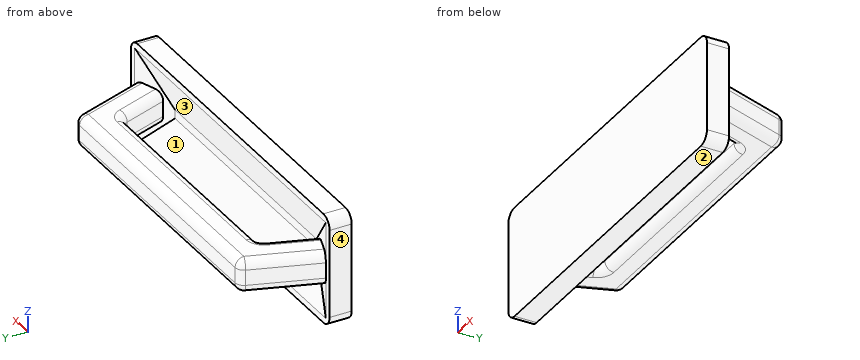
```python
from build123d import *

# Parameters (mm, degrees)
SKETCH1_W                = 160
SKETCH1_H                = 50
BOSS_EXTRUDE1_DEPTH      = 10
SHELL3_T                 = -3
FILLET1_R                = 5
CHAMFER1_SIZE            = 7
CHAMFER1_SIZE_2          = 20
BOSS_EXTRUDE2_DEPTH      = 7.5
BOSS_EXTRUDE2_DEPTH_BACK = 7.5
FILLET2_R                = 4


with BuildPart() as part:
    # Sketch1 → Boss-Extrude1 (new body)
    with BuildSketch(Plane(origin=(0, 0, 0), x_dir=(1, 0, 0), z_dir=(0, 1, 0))):
        Rectangle(SKETCH1_W, SKETCH1_H)
    extrude(amount=BOSS_EXTRUDE1_DEPTH)

    # Shell3
    shell3_openings = [part.faces().sort_by_distance(p)[0] for p in [
        (0, 10, 0),
    ]]
    offset(amount=SHELL3_T, openings=shell3_openings, kind=Kind.INTERSECTION)

    # Fillet1
    fillet1_edges = [part.edges().sort_by_distance(p)[0] for p in [
        (80, 5, 25),
        (-80, 5, 25),
        (-80, 5, -25),
        (80, 5, -25),
    ]]
    fillet(fillet1_edges, radius=FILLET1_R)

    # Chamfer1
    # the kernel refuses this chamfer: 20, 7 mm, written as the material it adds along each edge
    with BuildSketch(Plane(origin=(-77, 3, 22), x_dir=(0, 0.9946410899892074, 0.10338811394488961), z_dir=(1, 0, 0))) as chamfer1_piece_1_section:
        Polygon((CHAMFER1_SIZE * 0.994641089989, -CHAMFER1_SIZE * 0.103388113945), (-CHAMFER1_SIZE_2 * 0.103388113945, -CHAMFER1_SIZE_2 * 0.994641089989), (0, 0), align=None)
    chamfer1_piece_1 = extrude(amount=154, mode=Mode.PRIVATE)
    chamfer1_piece_1 = split(chamfer1_piece_1, bisect_by=Plane(origin=(0, 10, 15.125023974), z_dir=(0, -1, 0)), keep=Keep.TOP, mode=Mode.PRIVATE)
    add(chamfer1_piece_1)
    with BuildSketch(Plane(origin=(-77, 3, -22), x_dir=(-0.10338811394489059, 0.9946410899892072, 0), z_dir=(0, 0, 1))) as chamfer1_piece_2_section:
        Polygon((CHAMFER1_SIZE * 0.994641089989, -CHAMFER1_SIZE * 0.103388113945), (-CHAMFER1_SIZE_2 * 0.103388113945, -CHAMFER1_SIZE_2 * 0.994641089989), (0, 0), align=None)
    chamfer1_piece_2 = extrude(amount=44, mode=Mode.PRIVATE)
    chamfer1_piece_2 = split(chamfer1_piece_2, bisect_by=Plane(origin=(-70.125023974, 10, 0), z_dir=(0, -1, 0)), keep=Keep.TOP, mode=Mode.PRIVATE)
    add(chamfer1_piece_2)
    with BuildSketch(Plane(origin=(77, 3, -22), x_dir=(0, 0.9946410899892074, -0.10338811394488961), z_dir=(-1, 0, 0))) as chamfer1_piece_3_section:
        Polygon((CHAMFER1_SIZE * 0.994641089989, -CHAMFER1_SIZE * 0.103388113945), (-CHAMFER1_SIZE_2 * 0.103388113945, -CHAMFER1_SIZE_2 * 0.994641089989), (0, 0), align=None)
    chamfer1_piece_3 = extrude(amount=154, mode=Mode.PRIVATE)
    chamfer1_piece_3 = split(chamfer1_piece_3, bisect_by=Plane(origin=(0, 10, -15.125023974), z_dir=(0, -1, 0)), keep=Keep.TOP, mode=Mode.PRIVATE)
    add(chamfer1_piece_3)
    with BuildSketch(Plane(origin=(77, 3, 22), x_dir=(0.10338811394489059, 0.9946410899892072, 0), z_dir=(0, 0, -1))) as chamfer1_piece_4_section:
        Polygon((CHAMFER1_SIZE * 0.994641089989, -CHAMFER1_SIZE * 0.103388113945), (-CHAMFER1_SIZE_2 * 0.103388113945, -CHAMFER1_SIZE_2 * 0.994641089989), (0, 0), align=None)
    chamfer1_piece_4 = extrude(amount=44, mode=Mode.PRIVATE)
    chamfer1_piece_4 = split(chamfer1_piece_4, bisect_by=Plane(origin=(70.125023974, 10, 0), z_dir=(0, -1, 0)), keep=Keep.TOP, mode=Mode.PRIVATE)
    add(chamfer1_piece_4)

    # Sketch2 → Boss-Extrude2 (add, two sides: drawn at the far end of the back side and taken through both)
    with BuildSketch(Plane.XY.offset(-BOSS_EXTRUDE2_DEPTH_BACK)):
        Polygon((-65.45, 43), (-77, 10), (-62.842124655, 5.044743629), (-54.807784925, 28), (54.807784925, 28), (62.842124655, 5.044743629), (77, 10), (65.45, 43), align=None)
    extrude(amount=BOSS_EXTRUDE2_DEPTH + BOSS_EXTRUDE2_DEPTH_BACK)

    # Fillet2
    fillet2_edges = [part.edges().sort_by_distance(p)[0] for p in [
        (54.807784925, 28, 0),
        (0, 28, -7.5),
        (-54.807784925, 28, 0),
        (-58.82495479, 16.522371815, -7.5),
        (-71.225, 26.5, 7.5),
        (-65.45, 43, 0),
        (0, 43, 7.5),
        (65.45, 43, 0),
        (71.225, 26.5, 7.5),
        (58.82495479, 16.522371815, -7.5),
        (-71.225, 26.5, -7.5),
        (0, 43, -7.5),
        (71.225, 26.5, -7.5),
        (0, 28, 7.5),
        (58.82495479, 16.522371815, 7.5),
        (-58.82495479, 16.522371815, 7.5),
    ]]
    fillet(fillet2_edges, radius=FILLET2_R)


solid = part.part
```
Read the model definition and answer for the solid it produces. Units are mm, in the model's axes. Face numbers are marked on the shaded views. Give positions to 0.01 mm unless a question says otherwise; leave off trailing zeros. Order: outer loops, then holes, each group sorted by start corner. A loop starts at its lowest first (then second) coordinate and runs counter-clockwise, first axis right, second up. Notation, with made-up numbers: (10, 46) -> (17, 46) arc R18 cw to (17, 71) -> close; hole circle Ø2 at (3, 33). An arc over 180 degrees is marked (long way). Write item = value, one per line.
1. A cutting plane is placed at D-D, the plane z = -13. Write down the section's boundary in (x, y), and give its area (3 significant figures).
Numbers:
outline = (-80, 0) -> (80, 0) -> (80, 10) -> (77, 10) -> (68, 6.85) -> (-68, 6.85) -> (-77, 10) -> (-80, 10) -> close
area = 1,140 mm²
2. The mould has two halves that part along X. Classify the marked faces 1, 2, 3 and 4: +X half, -X half, draft (parallel to the pull), parting line (faces both ways), or undercut.
Numbers:
face_1 = undercut
face_2 = draft
face_3 = undercut
face_4 = -X half
3. Given pin 1 (4 mm diameter, centred on x = -42.5, z = -11, fed in from +Y); pin 2 (10 mm diameter, centred on x = 62, y = 18.5, fed in from +Z); pin 3 (16.5 mm diameter, centred on x = -27, y = 26, fed in from -Z), each flat-ended and moving along its own axis, determine where each tip first touches the part or whether it passes through.
Numbers:
pin_1 = 6.85
pin_2 = 7.5
pin_3 = -7.5
4. A cutting plane is placed at C-C, the plane z = 6. Write down the section's boundary in (x, y) (1 decimal).
Numbers:
outline = (-80, 0) -> (80, 0) -> (80, 10) -> (77, 10) -> (76.2, 9.7) -> (65.6, 40) arc R3.1 ccw to (62.6, 42.1) -> (-62.6, 42.1) arc R3.1 ccw to (-65.6, 40) -> (-76.2, 9.7) -> (-77, 10) -> (-80, 10) -> close; hole (-63.7, 5.3) -> (-61, 4.4) -> (61, 4.4) -> (63.7, 5.3) -> (56.6, 25.6) arc R4.9 ccw to (52, 28.9) -> (-52, 28.9) arc R4.9 ccw to (-56.6, 25.6) -> close
5. A cutting plane is placed at B-B, the plane z = 18. Write down the section's boundary in (x, y).
Numbers:
outline = (-80, 0) -> (80, 0) -> (80, 10) -> (77, 10) -> (73, 8.6) -> (-73, 8.6) -> (-77, 10) -> (-80, 10) -> close
6. Straight lines are drawn through the part: line 1 along Z through (x, y) = (-29, 37); line 2 along Y through (x, z) = (23.5, -2.5) (3 decimals); line 3 along X through (y, z) = (18.5, -6.5). For each, find the intervals that lie inside material, in ascending order.
Numbers:
line_1 = -7.5 to 7.5
line_2 = 0 to 3.175, 28 to 43
line_3 = -72.59 to -59.57, 59.57 to 72.59
7. A cutting plane is placed at A-A, the plane x = -26.5. Write down the section's boundary in (y, z), and give its area (3 significant figures).
Numbers:
outline = (0, -25) -> (10, -25) -> (10, -22) -> (3, -2) -> (3, 2) -> (10, 22) -> (10, 25) -> (0, 25) -> close; (28, -3.5) arc R4 ccw to (32, -7.5) -> (39, -7.5) arc R4 ccw to (43, -3.5) -> (43, 3.5) arc R4 ccw to (39, 7.5) -> (32, 7.5) arc R4 ccw to (28, 3.5) -> close
area = 543 mm²
